Autodesk Inventor part; units mm, degrees
ref_plane "YZ Plane" through (0, 0, 0) normal (1, 0, 0) x (0, 1, 0)
ref_plane "XZ Plane" through (0, 0, 0) normal (0, 1, 0) x (-1, 0, 0)
ref_plane "XY Plane" through (0, 0, 0) normal (0, 0, 1) x (1, 0, 0)
sketch "Sketch1" plane through (0, 0, 0) normal (0, 0, 1) x (1, 0, 0)
  point P0 (0, 0)
sketch "Sketch2" plane through (0, 0, 0) normal (0, 0, 1) x (1, 0, 0)
  line L0 (0, 0) -> (10.9474, 0)
  line L1 (10.9474, 0) -> (10.9474, 10.9728)
  line L2 (10.9474, 10.9728) -> (0, 10.9728)
  line L3 (0, 10.9728) -> (0, 0)
  dimension "d0" = 10.9474
  dimension "d1" = 10.9728
extrude "Extrusion1" add sketch "Sketch2" along normal blind 1.016
sketch "Sketch3" plane through (0, 0, 1.016) normal (0, 0, 1) x (1, 0, 0)
  line L0 (0, 0) -> (10.9474, 0)
  line L1 (2.2167, 0) -> (6.4763, 0)
  line L2 (6.4763, 0) -> (6.4763, 2.2384)
  line L3 (6.4763, 2.2384) -> (2.2167, 2.2384)
  line L4 (2.2167, 2.2384) -> (2.2167, 0)
  line L5 (8.5191, 6.2372) -> (9.3015, 6.2372)
  line L6 (9.3015, 6.2372) -> (9.3015, 5.7591)
  line L7 (9.3015, 5.7591) -> (8.5191, 5.7591)
  line L8 (8.5191, 5.7591) -> (8.5191, 6.2372)
extrude "Extrusion2" cut sketch "Sketch3" against normal blind 1.016 contours L4 L3 L2 L0
sketch "Sketch4" plane through (0, 0, 1.016) normal (0, 0, 1) x (1, 0, 0)
  line L0 (8.4757, 6.2372) -> (9.4319, 6.2372)
  line L1 (9.4319, 6.2372) -> (9.4319, 5.846)
  line L2 (9.4319, 5.846) -> (8.4757, 5.846)
  line L3 (8.4757, 5.846) -> (8.4757, 6.2372)
  point P0 (0, 0)
extrude "Extrusion3" cut sketch "Sketch4" against normal blind 1.016
properties part number "front"
Model file for the job. Use its own axes, mm. A direction names the side the tool comes from. Round coordinates to 2 decimals unless told otherwise and drop trailing zeros. Loops run counter-clockwise (first coordinate to the right, second up) from the corner with the lowest first, then second, coordinate; pieces in that order, holes last. Notation, with made-up numbers: (-37, 7) - (-30, 7) arc R21 cw to (-30, 29) - close; hole circle Ø6 at (70, 16). An arc over 180 degrees is marked (long way). Write each question's results on one line, items separated by ' | '.
(1) Saw through at C-C, the plane x = 5.5. List the corners of the cut face in (y, z), then the cut area to 3 significant figures.
Answer below:
outline: (2.24, 0) - (10.97, 0) - (10.97, 1.02) - (2.24, 1.02) - close | area: 8.87 mm^2
(2) Saw through at B-B, the plane z = 0.6. List the corners of the cut face in (x, y), then the cut area to 3 significant figures.
Answer below:
outline: (0, 0) - (2.22, 0) - (2.22, 2.24) - (6.48, 2.24) - (6.48, 0) - (10.95, 0) - (10.95, 10.97) - (0, 10.97) - close; hole (8.48, 5.85) - (9.43, 5.85) - (9.43, 6.24) - (8.48, 6.24) - close | area: 110 mm^2
(3) Mould opens along X. For faces 4 (the flat face through (1.1, 0, 0.5)), 5 (the flat face through (10.947, 5.4, 0.5)), 6 (the flat face through (4.4, 2.238, 0.5)) say: released by +X, released by -X, zero draft, split by the parting line, or undercut.
Answer below:
face 4: zero draft | face 5: released by +X | face 6: undercut
(4) Wall check: L1, parallel to X at y = 1.5, z = 0.2; L2, parallel to Y at x = 2.25, z = 0.4. Give the ranges that are in metal, low to high.
Answer below:
L1: x = 0 to 2.22, 6.48 to 10.95 | L2: y = 2.24 to 10.97
(5) Saw through at A-A, the plane y = 1.5. List the corners of the cut face in (x, z).
Answer below:
outline: (0, 0) - (2.22, 0) - (2.22, 1.02) - (0, 1.02) - close; (6.48, 0) - (10.95, 0) - (10.95, 1.02) - (6.48, 1.02) - close
(6) 3-axis set-ups, long thin cutter, end or side, ignore diameter. For faces 1 (the flat face through (8.9, 6.237, 0.5)), 2 (the flat face through (2.217, 1.1, 0.5)), 3 (the flat face through (8.7, 0, 0.5)): which of +Z, -Z, +X, -X, +Y, -Y reach the whole face in a straight line?
Answer below:
face 1: +Z, -Z | face 2: +Z, -Z, -Y | face 3: +Z, -Z, +X, -X, -Y
